Geometry check sheet. Reference: the model listing, model coordinates, mm. A direction names the side the tool comes from. Coordinates: 2 decimals unless noted, no trailing zeros. Order: outer loops, then holes, each group sorted by start corner. A loop starts at its lowest first (then second) coordinate and runs counter-clockwise, first axis right, second up. Notation, with made-up numbers: (21, 45.25) - (38, 45.25) arc R10 ccw to (38, 64.25) - close; hole circle Ø3 at (-24.5, 76). An arc over 180 degrees is marked (long way). Put each result on its own line as item: value.
from build123d import *

# Parameters (mm, degrees)
F0_W     = 59.4606287777
F0_H     = 47.7610453963
F1_DEPTH = 25
F2_T     = -1
F3_R     = 5


with BuildPart() as f1:
    # F0 (on Front) → F1 (new body)
    with BuildSketch(Plane.XZ):
        with Locations((29.7303143889, 23.8805226982)):
            Rectangle(F0_W, F0_H)
        Polygon((28.3158866396, 45.8665414289), (42.3948997325, 30.5626016077), (32.1906423503, 12.443486977), (11.8050513651, 16.5491981105), (9.4103206379, 37.2057817696), align=None, mode=Mode.SUBTRACT)
    extrude(amount=F1_DEPTH)

    # F2
    f2_openings = [f1.faces().sort_by_distance(p)[0] for p in [
        (0.762672, -25, 23.880523),
    ]]
    offset(amount=F2_T, openings=f2_openings, kind=Kind.INTERSECTION)

    # F3
    f3_edges = [f1.edges().sort_by_distance(p)[0] for p in [
        (58.460629, -13, 46.761045),
        (59.460629, -12.5, 47.761045),
    ]]
    fillet(f3_edges, radius=F3_R)


solid = f1.part
Q1. Thickness scan on L1, parallel to Z at x = 5, y = -17; L2, parallel to Z at x = 24, y = -16.5; L3, parallel to X at y = -1.75, z = 5. Record the ranges inside material, lowest first. Write a range as [from, to].
Answer block:
L1: z = [0, 1], [46.76, 47.76]
L2: z = [0, 1], [13.07, 14.09], [43.89, 44.99], [46.76, 47.76]
L3: x = [0, 1], [58.46, 59.46]
Q2. Draft check along Z on faces 1 (the cylindrical face through (57.957, -12.675, 46.335)), 2 (the flat face through (29, -12, 0)), 3 (the flat face through (41, -13, 46.761)). Enter one of: pulls with the +Z half, pulls with the -Z half, needs draft (parallel to the pull), parting line crosses it, or undercut.
Answer block:
face 1: pulls with the +Z half
face 2: pulls with the -Z half
face 3: undercut
Q3. Section check C-C on x = 14.5. Record the boundary of the cut face in (y, z), then the cut area to 3 significant figures.
Answer block:
outline: (-25, 0) - (0, 0) - (0, 16.01) - (-25, 16.01) - (-25, 14.99) - (-1, 14.99) - (-1, 1) - (-25, 1) - close; (-25, 39.54) - (0, 39.54) - (0, 47.76) - (-25, 47.76) - (-25, 46.76) - (-1, 46.76) - (-1, 40.64) - (-25, 40.64) - close
area: 123 mm^2
Q4. Access from +Z, -Z, +X, -X, +Y, -Y to the whole of each face (thin tool, end or side, straight path). Record for faces 4 (the flat face through (37.364, -12.325, 21.63)), 5 (the flat face through (17.964, -12.832, 42.224)), 6 (the flat face through (16, -25, 15)).
Answer block:
face 4: +Y, -Y
face 5: -Y
face 6: +Z, -Z, +X, -X, -Y
Q5. Section check A-A on y = -19. Record the boundary of the cut face in (x, z), then the cut area to 3 significant figures.
Answer block:
outline: (0, 0) - (59.46, 0) - (59.46, 42.76) arc R5 ccw to (54.46, 47.76) - (0, 47.76) - close; hole (1, 1) - (58.46, 1) - (58.46, 41.76) arc R5 ccw to (53.46, 46.76) - (28.85, 46.76) - (43.62, 30.7) - (32.71, 11.32) - (10.9, 15.71) - (8.33, 37.81) - (27.87, 46.76) - (1, 46.76) - close; hole (9.41, 37.21) - (11.81, 16.55) - (32.19, 12.44) - (42.39, 30.56) - (28.32, 45.87) - close
area: 318 mm^2
Q6. Section check D-D on x = 48. Record the boundary of the cut face in (y, z).
Answer block:
outline: (-25, 0) - (0, 0) - (0, 47.76) - (-25, 47.76) - (-25, 46.76) - (-1, 46.76) - (-1, 1) - (-25, 1) - close
Q7. Section check B-B on z = 34. Record the boundary of the cut face in (x, y), then the cut area to 3 significant figures.
Answer block:
outline: (0, -25) - (1, -25) - (1, -1) - (8.78, -1) - (8.78, -25) - (9.78, -25) - (9.78, 0) - (0, 0) - close; (39.23, -25) - (40.59, -25) - (40.59, -1) - (58.46, -1) - (58.46, -25) - (59.46, -25) - (59.46, 0) - (39.23, 0) - close
area: 135 mm^2
